Input: part model. Units: mm. Frame: model coordinates. A direction names the side the tool comes from. Coordinates: 2 decimals unless noted, no trailing zeros. Order: outer loops, then holes, each group sorted by start corner. A loop starts at its lowest first (then second) coordinate and runs counter-clockwise, first axis right, second up. Notation, with made-up numbers: M 89,34.5 L 143,34.5 A31 ccw 143,58.5 Z; hole C 74,31.25 d6. An arc over 180 degrees is marked long. Answer in a Markdown table with one row per item.
from build123d import *

# Parameters (mm, degrees)
F0_R     = 29.845
F0_R_2   = 23.495
F1_DEPTH = 3.175
F2_R     = 26.67
F2_R_2   = 23.495
F3_DEPTH = 66.1543
F4_R     = 26.67
F4_R_2   = 2.2479
F5_DEPTH = 3.175


with BuildPart() as f1:
    # F0 (on Top) → F1 (new body)
    with BuildSketch(Plane.XY):
        Circle(F0_R)
        Circle(F0_R_2, mode=Mode.SUBTRACT)
    extrude(amount=F1_DEPTH)

    # F2 (on face) → F3 (join)
    with BuildSketch(Plane.XY.offset(3.175)):
        Circle(F2_R)
        Circle(F2_R_2, mode=Mode.SUBTRACT)
    extrude(amount=F3_DEPTH)

    # F4 (on face) → F5 (join)
    with BuildSketch(Plane.XY.offset(69.3293)):
        Circle(F4_R)
        with Locations((-16.910229, -9.763125)):
            Circle(F4_R_2, mode=Mode.SUBTRACT)
        with Locations((16.910229, -9.763125)):
            Circle(F4_R_2, mode=Mode.SUBTRACT)
        with Locations((0, 19.52625)):
            Circle(F4_R_2, mode=Mode.SUBTRACT)
    extrude(amount=F5_DEPTH)


solid = f1.part
1) Mould query, pull axis Y, two halves, no side actions, for faces 1 (the face through (9, -22, 0)), 2 (the face through (14.665, -9.664, 70.895)), 3 (the face through (28.47, 8.96, 1.57)). Classes: +Y half, -Y half, draft (parallel to the pull), parting line (faces both ways), or undercut.
Resolved:
| item | result |
|---|---|
| face 1 | draft |
| face 2 | undercut |
| face 3 | parting line |
2) Cut plane C-C, the plane z = 49. Output: boundary loops of the cut face in (x, y) (3 decimals), and give its area (3 significant figures).
Resolved:
| item | result |
|---|---|
| outline | C 0,0 d53.34; hole C 0,0 d46.99 |
| area | 500 mm2 |
3) Material intervals for probe 1 along Y at (x, z) = (0, 17) (3 decimals); probe 2 along Y at (x, z) = (8, 60.5); probe 3 along Z at (x, y) = (-7, -12), sorted ascending.
Resolved:
| item | result |
|---|---|
| probe 1 | y = -26.67 to -23.495, 23.495 to 26.67 |
| probe 2 | y = -25.44 to -22.09, 22.09 to 25.44 |
| probe 3 | z = 69.33 to 72.5 |
4) Cut plane A-A, the plane x = 0. Output: boundary loops of the cut face in (y, z) (3 decimals), and give its area (3 significant figures).
Resolved:
| item | result |
|---|---|
| outline | M -29.845,0 L -23.495,0 L -23.495,69.329 L 17.278,69.329 L 17.278,72.504 L -26.67,72.504 L -26.67,3.175 L -29.845,3.175 Z; M 21.774,69.329 L 23.495,69.329 L 23.495,0 L 29.845,0 L 29.845,3.175 L 26.67,3.175 L 26.67,72.504 L 21.774,72.504 Z |
| area | 615 mm2 |
5) Cut plane D-D, the plane x = 12.5. Output: boundary loops of the cut face in (y, z) (3 decimals).
Resolved:
| item | result |
|---|---|
| outline | M -27.101,0 L -19.894,0 L -19.894,69.329 L 19.894,69.329 L 19.894,0 L 27.101,0 L 27.101,3.175 L 23.559,3.175 L 23.559,72.504 L -23.559,72.504 L -23.559,3.175 L -27.101,3.175 Z |
6) Contact query for flat-ended pins moving along their axis: pin 1 (12 mm diameter, centred on x = -19, z = 13.5, fed in from +Y); pin 2 (12 mm diameter, centred on y = 11.5, z = 17, fed in from +X); pin 3 (10 mm diameter, centred on y = 16, z = 12.5, fed in from -X). Output: stop coordinate, or through.
Resolved:
| item | result |
|---|---|
| pin 1 | stops at y = 23.29 |
| pin 2 | stops at x = 26.1 |
| pin 3 | stops at x = -24.3 |
7) Cut plane B-B, the plane y = -3. Output: boundary loops of the cut face in (x, z) (3 decimals).
Resolved:
| item | result |
|---|---|
| outline | M -29.694,0 L -23.303,0 L -23.303,69.329 L 23.303,69.329 L 23.303,0 L 29.694,0 L 29.694,3.175 L 26.501,3.175 L 26.501,72.504 L -26.501,72.504 L -26.501,3.175 L -29.694,3.175 Z |
8) Reachability of faces 4 (the face through (0, 0, 72.504)), 5 (the face through (-5.093, -22.936, 34.179)), 6 (the face through (-22.2, -15.3, 3.175)) from +Z, -Z, +X, -X, +Y, -Y: full face, straight path, thin tool, end or side. Return the list, or none.
Resolved:
| item | result |
|---|---|
| face 4 | +Z, +X, -X, +Y, -Y |
| face 5 | -Z |
| face 6 | +Z |
